```python
from build123d import *

# Parameters (mm, degrees)
SKETCH_2_W          = 55.5
SKETCH_2_H          = 20
SKETCH_2_R          = 1.5
EXTRUDE_1_DEPTH     = 2
SKETCH_3_W          = 2
SKETCH_3_H          = 20
EXTRUDE_2_DEPTH     = 35
SKETCH_4_R          = 1.5
SKETCH_4_R_2        = 4
CUT_EXTRUDE_1_DEPTH = 65


with BuildPart() as part:
    # 스케치2 → 보스-돌출1 (new body)
    with BuildSketch(Plane(origin=(0, 0, 0), x_dir=(1, 0, 0), z_dir=(0, 1, 0))):
        Rectangle(SKETCH_2_W, SKETCH_2_H)
        with Locations(Location((-15, 5, 0), (0, 0, 270))):
            Circle(SKETCH_2_R, mode=Mode.SUBTRACT)
        with Locations(Location((-5, 5, 0), (0, 0, 270))):
            Circle(SKETCH_2_R, mode=Mode.SUBTRACT)
        with Locations(Location((-15, -5, 0), (0, 0, 270))):
            Circle(SKETCH_2_R, mode=Mode.SUBTRACT)
        with Locations(Location((-5, -5, 0), (0, 0, 270))):
            Circle(SKETCH_2_R, mode=Mode.SUBTRACT)
        with Locations(Location((15, -5, 0), (0, 0, 90))):
            Circle(SKETCH_2_R, mode=Mode.SUBTRACT)
        with Locations(Location((5, -5, 0), (0, 0, 90))):
            Circle(SKETCH_2_R, mode=Mode.SUBTRACT)
        with Locations(Location((5, 5, 0), (0, 0, 90))):
            Circle(SKETCH_2_R, mode=Mode.SUBTRACT)
        with Locations(Location((15, 5, 0), (0, 0, 90))):
            Circle(SKETCH_2_R, mode=Mode.SUBTRACT)
    extrude(amount=EXTRUDE_1_DEPTH)

    # 스케치3 → 보스-돌출2 (add)
    with BuildSketch(Plane(origin=(0, 2, 0), x_dir=(1, 0, 0), z_dir=(0, 1, 0))):
        with Locations((-26.75, 0)):
            Rectangle(SKETCH_3_W, SKETCH_3_H)
        with Locations((26.75, 0)):
            Rectangle(SKETCH_3_W, SKETCH_3_H)
    extrude(amount=EXTRUDE_2_DEPTH)

    # 스케치4 → 컷-돌출1 (cut)
    with BuildSketch(Plane(origin=(27.75, 0, 0), x_dir=(0, 0, -1), z_dir=(1, 0, 0))):
        with BuildLine():
            Line((-10, 37), (-10, 27))
            ThreePointArc((-10, 27), (-7.071067815, 34.071067809), (-9e-09, 37))
            Line((-9e-09, 37), (-10, 37))
        make_face()
        with BuildLine():
            Line((10, 37), (-9e-09, 37))
            ThreePointArc((-9e-09, 37), (7.071067809, 34.071067815), (10, 27))
            Line((10, 27), (10, 37))
        make_face()
        with Locations((7.07, 27)):
            Circle(SKETCH_4_R)
        with Locations((0, 27)):
            Circle(SKETCH_4_R_2)
        with Locations((0, 34.07)):
            Circle(SKETCH_4_R)
        with Locations((4.999244943, 22.000755057)):
            Circle(SKETCH_4_R)
        with Locations((0, 19.93)):
            Circle(SKETCH_4_R)
        with Locations((-4.999244943, 22.000755057)):
            Circle(SKETCH_4_R)
        with Locations((-7.07, 27)):
            Circle(SKETCH_4_R)
    extrude(amount=-CUT_EXTRUDE_1_DEPTH, mode=Mode.SUBTRACT)


solid = part.part
```
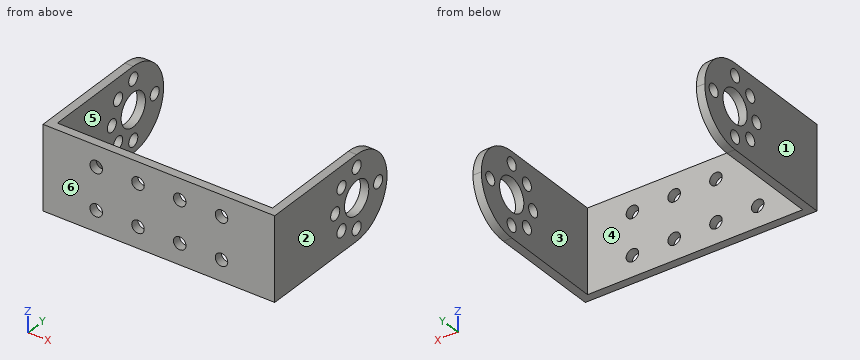
Could you check a few things on this model? Use its own coordinates, in mm. Face numbers are marked on the shaded views. A direction names the side the tool comes from. Coordinates: 2 decimals unless noted, no trailing zeros. Order: outer loops, then holes, each group sorted by start corner. A loop starts at its lowest first (then second) coordinate and runs counter-clockwise, first axis right, second up. Notation, with made-up numbers: M 19.5,-10 L 58.5,-10 A7 cw 58.5,-1 Z; hole C 6.5,-16.75 d1. An arc over 180 degrees is marked long. Use one line per item in the form item = value. Start each with the question number.
1. We'd pull the mould along X, two halves only. Please class the marked faces 1, 2, 3 and 4: +X half, -X half, draft (parallel to the pull), parting line (faces both ways), or undercut.
2. For pin 1 (4 mm diameter, centred on x = 21, z = 1, fed in from +Y), with a flat end and sliding along its axis, tell me the tip position at first contact or that it passes through.
3. Suppose I cut it at B-B on y = 17. Write out the boundary of the cut face in (x, z), then the cut area to 3 significant figures.
4. On a 3-axis mill with a long thin cutter (end or side, diameter ignored), from which of +Z, -Z, +X, -X, +Y, -Y can I reach the whole of each face in a straight line? I mean the marked faces 5 and 6. Say none if no direction works.
5. Suppose I cut it at A-A on x = -15. Write out the boundary of the cut face in (y, z).
6. Please list where these lines run through material, in increasing order: line 1 (Z direction, x = 5, y = 1.1); line 2 (X direction, y = 1.5, z = -5); line 3 (X direction, y = 11, z = -3.25).
7. Suppose I cut it at C-C on z = 4.75. Count the separate pieces of the cut face and the enclosed holes in it, then the cut area to 3 significant figures.
8. Suppose I cut it at D-D on z = -7.07. Write out the boundary of the cut face in (x, y), then the cut area to 3 significant figures.
Geometry says:
q1.face_1 = -X half
q1.face_2 = +X half
q1.face_3 = undercut
q1.face_4 = undercut
q2.pin_1 = 2
q3.outline = M -27.75,-10 L -25.75,-10 L -25.75,10 L -27.75,10 Z; M 25.75,-10 L 27.75,-10 L 27.75,10 L 25.75,10 Z
q3.area = 80.0 mm^2
q4.face_5 = +Z, -Z, +Y
q4.face_6 = +Z, -Z, +X, -X, -Y
q5.outline = M 0,-10 L 2,-10 L 2,-6.5 L 0,-6.5 Z; M 0,-3.5 L 2,-3.5 L 2,3.5 L 0,3.5 Z; M 0,6.5 L 2,6.5 L 2,10 L 0,10 Z
q6.line_1 = -10 to -6.5, -3.5 to 3.5, 6.5 to 10
q6.line_2 = -27.75 to -16.5, -13.5 to -6.5, -3.5 to 3.5, 6.5 to 13.5, 16.5 to 27.75
q6.line_3 = -27.75 to -25.75, 25.75 to 27.75
q7.separate_pieces = 7
q7.enclosed_holes = 0
q7.area = 211 mm^2
q8.outline = M -27.75,0 L 27.75,0 L 27.75,25.5 L 25.75,25.5 L 25.75,2 L -25.75,2 L -25.75,25.5 L -27.75,25.5 Z; M -27.75,28.5 L -25.75,28.5 L -25.75,34.07 L -27.75,34.07 Z; M 25.75,28.5 L 27.75,28.5 L 27.75,34.07 L 25.75,34.07 Z
q8.area = 227 mm^2
